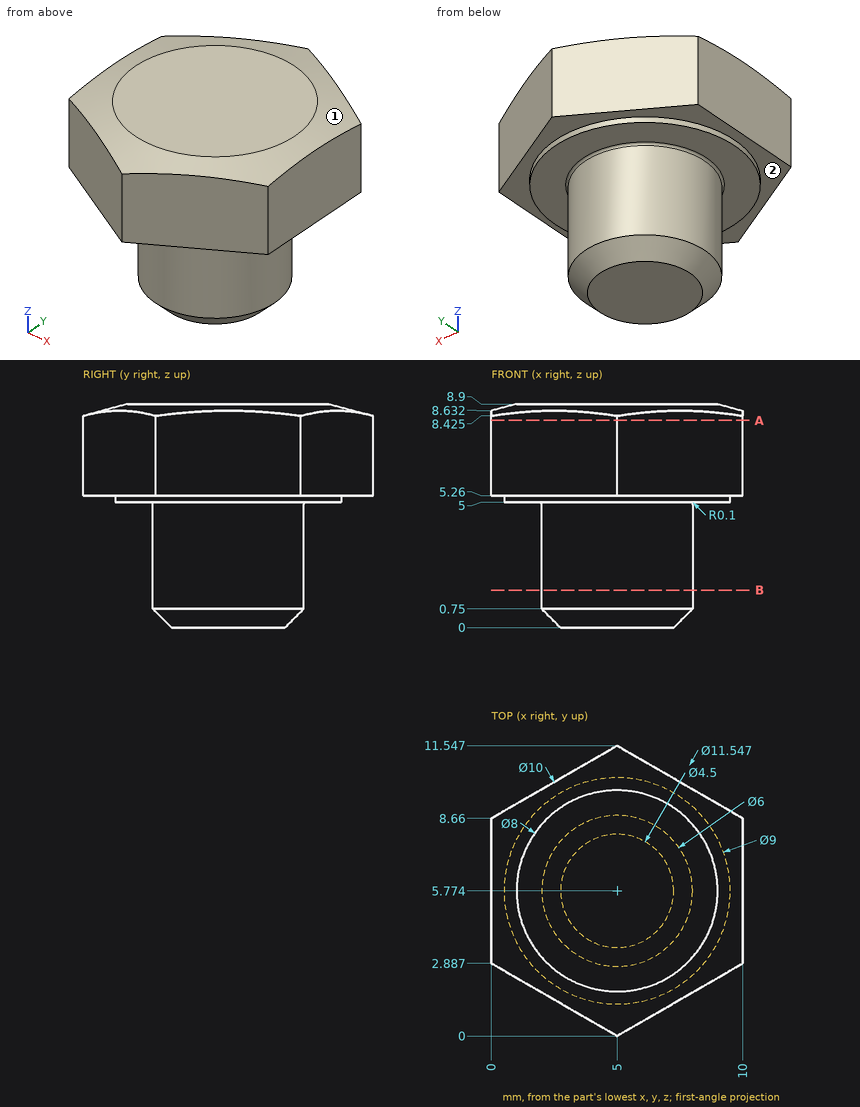
Answer from the drawing. Dimensions are ordinates in mm from the lowest x, y and z of the part. A direction names the side the tool comes from. Coordinates: 2 decimals unless noted, no trailing zeros. Order: outer loops, then holes, each group sorted by start corner. A loop starts at its lowest first (then second) coordinate and runs counter-clockwise, first axis right, second up. Notation, with made-up numbers: (68.25, 89.25) -> (120.25, 89.25) arc R15 ccw to (120.25, 118.25) -> close; hole circle Ø3 at (36, 87). An arc over 180 degrees is marked (long way). Answer as a JSON object with one key per item and string values.
1) Consider line 1 along Z through (x, y) = (4.75, 2.5); line 2 along Z through (x, y) = (6.5, 1); line 3 along Y through (x, z) = (5.75, 3.5). Determine where each line is inside the solid, lowest interval first. Write a range as from..to.
Model answer:
{"line 1": "z = 5..8.9", "line 2": "z = 5.26..8.63", "line 3": "y = 2.87..8.68"}
2) A tool of negligible diameter and unlimited length cuts with its end or side. For the marked faces 1 and 2, from which of +Z, -Z, +X, -X, +Y, -Y can it reach the whole face along a straight path? Write none if from no direction.
Model answer:
{"face 1": "+Z", "face 2": "-Z"}
3) A cutting plane is placed at A-A, the plane z = 8.25. Determine the outline of the cut face in (x, y), plus the area to 3 significant figures.
Model answer:
{"outline": "(0, 2.89) -> (5, 0) -> (10, 2.89) -> (10, 8.66) -> (5, 11.55) -> (0, 8.66) -> close", "area": "86.6 mm²"}
4) Each of these flat-tipped pins is pushed along its axis until it touches: pin 1 (1 mm diameter, centred on y = 2, z = 7.5, fed in from -X); pin 2 (1 mm diameter, centred on x = 2.5, y = 4.5, fed in from -Z) (1 decimal); pin 3 (1.5 mm diameter, centred on x = 7.5, z = 2.5, fed in from -Y). Where does it stop, or does it pass through?
Model answer:
{"pin 1": "stops at x = 0.67", "pin 2": "stops at z = 0.1", "pin 3": "stops at y = 3.34"}
5) A cutting plane is placed at B-B, the plane z = 1.5. Determine the outline of the cut face in (x, y), plus the area to 3 significant figures.
Model answer:
{"outline": "circle Ø6 at (5, 5.77)", "area": "28.3 mm²"}
